The drawing under review shows one solid part. Ordinate dimensions are in mm from its lowest x, y, z. A direction names the side the tool comes from. Round coordinates to 2 decimals unless told otherwise and drop trailing zeros. Order: outer loops, then holes, each group sorted by start corner. A loop starts at its lowest first (then second) coordinate and runs counter-clockwise, first axis right, second up. Notation, with made-up numbers: (49, 58.5) -> (65, 58.5) arc R13 ccw to (65, 68.5) -> close; hole circle Ø4 at (14, -13.5). An arc over 180 degrees is marked (long way). Use a Markdown table: item, result. Add a question column.
1) Consider section C-C (y = 9). State the section outline as (x, z) points, plus the area to 3 significant figures.
2) Consider section A-A (z = 63). State the section outline as (x, y) points, plus the area to 3 significant figures.
3) Consider section B-B (x = 10). State the section outline as (y, z) points.
4) Machinability: for the marked faces 1 and 2, which of the approach directions +Z, -Z, +X, -X, +Y, -Y give a long, thin tool a straight path to every point of the face, cutting with its end or side? Answer none if there is none.
5) Draft analysis for pull direction X (two halves, no side actions). For the marked faces 3, 4 and 5, state which applies: pulls with the +X half, pulls with the -X half, needs draft (parallel to the pull), parting line crosses it, or undercut.
6) Wall thickness on line 1 along Y through (x, z) = (17.5, 45.5); line 2 along X through (y, z) = (9, 29): over which ranges is each line inside the solid? List them lowest first. Write a range as [from, to].
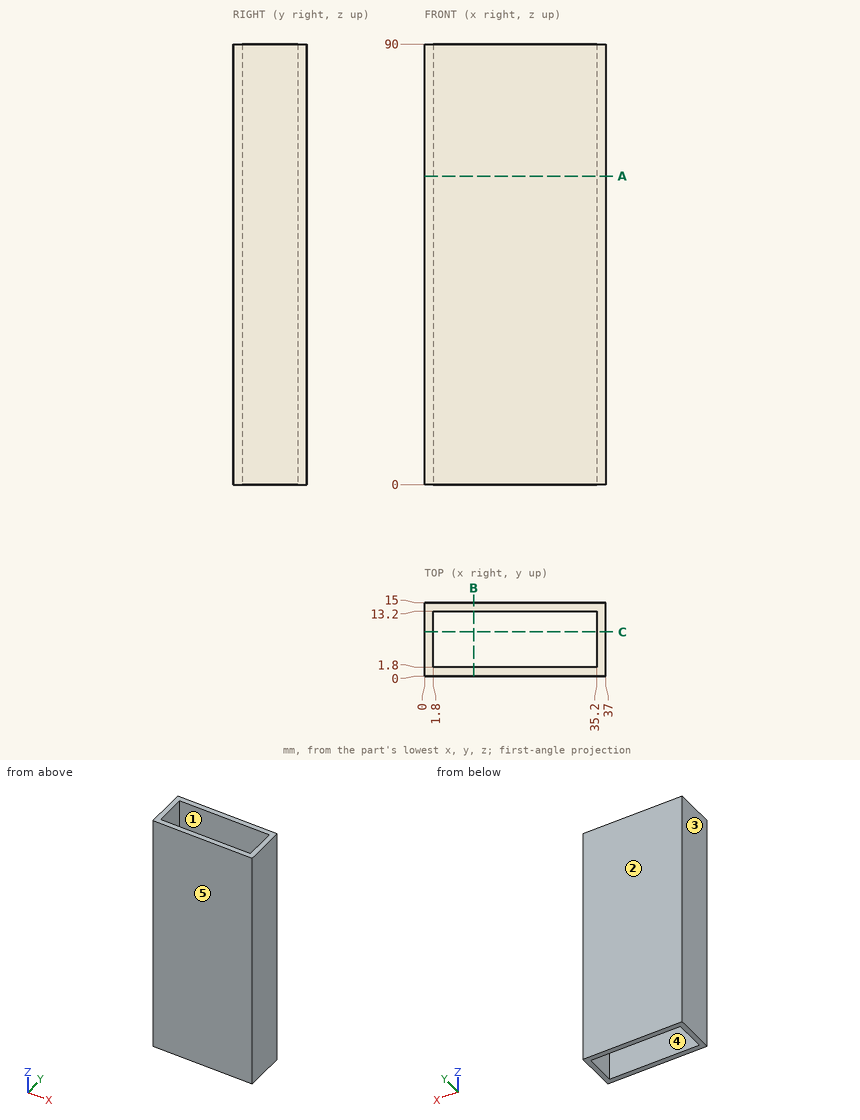
Results list:
| question | item | result |
|---|---|---|
| 1 | outline | (0, 0) -> (1.8, 0) -> (1.8, 90) -> (0, 90) -> close; (35.2, 0) -> (37, 0) -> (37, 90) -> (35.2, 90) -> close |
| 1 | area | 324 mm2 |
| 2 | outline | (0, 0) -> (37, 0) -> (37, 15) -> (0, 15) -> close; hole (1.8, 1.8) -> (35.2, 1.8) -> (35.2, 13.2) -> (1.8, 13.2) -> close |
| 2 | area | 174 mm2 |
| 3 | outline | (0, 0) -> (1.8, 0) -> (1.8, 90) -> (0, 90) -> close; (13.2, 0) -> (15, 0) -> (15, 90) -> (13.2, 90) -> close |
| 4 | face 1 | +Z, -Z |
| 4 | face 2 | +Z, -Z, +X, -X, +Y |
| 5 | face 3 | pulls with the -X half |
| 5 | face 4 | undercut |
| 5 | face 5 | needs draft |
| 6 | line 1 | [0, 1.8], [13.2, 15] |
| 6 | line 2 | [0, 1.8], [35.2, 37] |
